Study the drawing (mm; zero at the part's minimum x, y, z) and answer. A direction names the side the tool comes from. Give positions to 0.01 mm unless a question says otherwise; leave off trailing zeros. Write each loop counter-clockwise with the first axis right and the second up, starting at its lowest first coordinate (ties: lowest second). Pieces come first, ordered by that corner, then holes. Notation, with made-up numbers: (-19.75, 89) - (28.25, 89) arc R24 cw to (28.25, 126) - close; hole circle Ø1 at (-25.75, -3). An arc over 180 degrees is marked (long way). Answer in a Markdown table with one row per item. Add a question column.
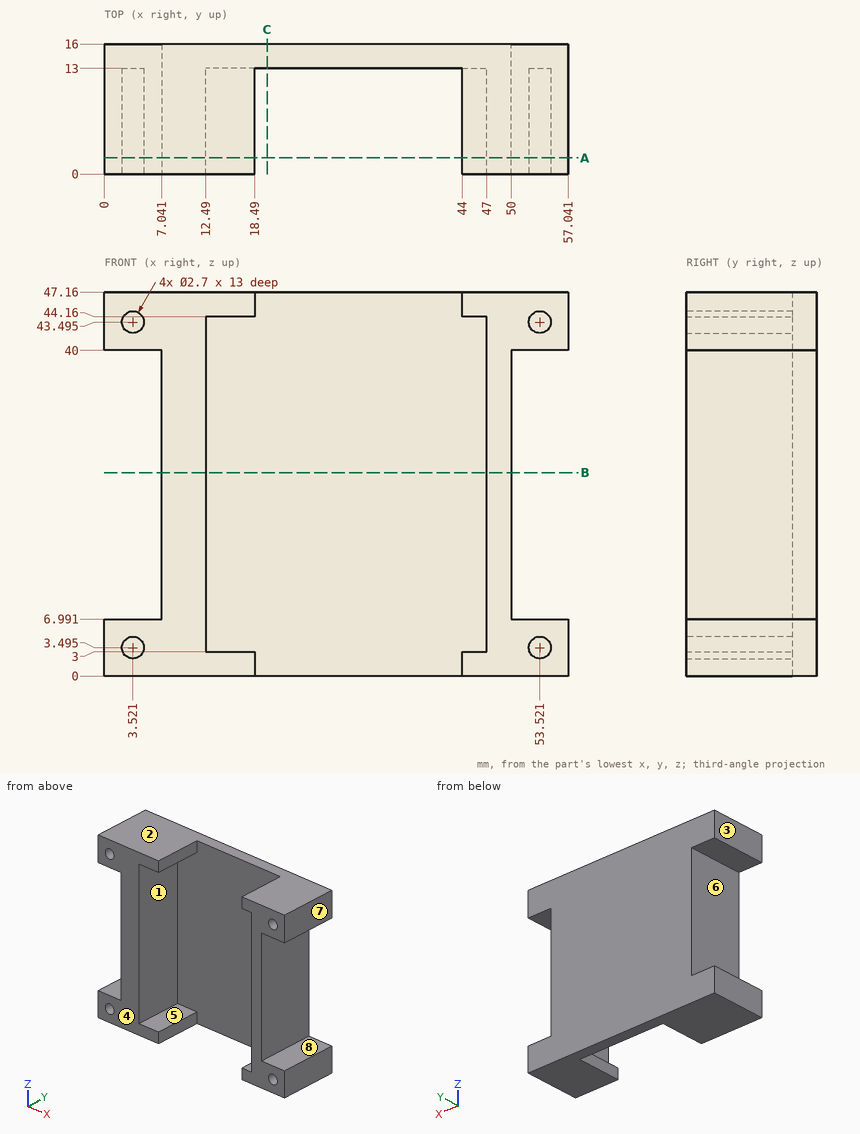
1. Straight lines are drawn through the part: L1, parallel to X at y = 8.75, z = 25; L2, parallel to Z at x = 6, y = 12; L3, parallel to X at y = 4, z = 2. For each, find the intervals that lie inside material, in ascending order. Write a range as [from, to].
2. Section B-B (z = 25) is taken. Give the vertices of the cut face in (x, y), and give its area (3 significant figures).
3. Section A-A (y = 2) is taken. State how many separate pieces and enclosed holes the cut face has, and give its area (3 significant figures).
4. Given pin 1 Ø8 at (y, z) = (5, 17) entering from -X; pin 2 Ø1.4 at (x, z) = (53.5, 44) entering from -Y; pin 3 Ø4 at (y, z) = (6, 20.5) entering from +X, each flat-ended and moving along its own axis, determine where each tip first touches the part or whether it passes through.
5. A tool of negligible diameter and unlimited length cuts with its end or side. For the marked faces 4, 5, 6, 7 and 8, from which of +Z, -Z, +X, -X, +Y, -Y can it reach the whole face along a straight path? Write none if from no direction.
6. Section C-C (x = 20) is taken. Give the vertices of the cut face in (y, z).
7. The mould has two halves that part along Z. Classify the marked faces 1, 2 and 3: +Z half, -Z half, draft (parallel to the pull), parting line (faces both ways), or undercut.
Geometry check:
| question | item | result |
|---|---|---|
| 1 | L1 | [7.04, 12.49], [47, 50] |
| 1 | L2 | [0, 6.99], [40, 47.16] |
| 1 | L3 | [0, 18.49], [44, 57.04] |
| 2 | outline | (7.04, 0) - (12.49, 0) - (12.49, 13) - (47, 13) - (47, 0) - (50, 0) - (50, 16) - (7.04, 16) - close |
| 2 | area | 239 mm² |
| 3 | separate pieces | 2 |
| 3 | enclosed holes | 4 |
| 3 | area | 629 mm² |
| 4 | pin 1 | x = 7.04 |
| 4 | pin 2 | y = 13 |
| 4 | pin 3 | x = 50 |
| 5 | face 4 | +Z, -Z, +X, -X, -Y |
| 5 | face 5 | -Y |
| 5 | face 6 | -X, +Y, -Y |
| 5 | face 7 | +Z, -Z, +X, +Y, -Y |
| 5 | face 8 | +X, +Y, -Y |
| 6 | outline | (13, 0) - (16, 0) - (16, 47.16) - (13, 47.16) - close |
| 7 | face 1 | undercut |
| 7 | face 2 | +Z half |
| 7 | face 3 | draft |
